The listing builds one solid part. Answer for the finished solid, in the listing's coordinates (mm). A direction names the side the tool comes from. Coordinates: 2 decimals unless noted, no trailing zeros. Write each loop counter-clockwise with the first axis right and the second up, starting at its lowest first coordinate (ties: lowest second). Pieces come first, ordered by that corner, then holes.
```python
from build123d import *

# Parameters (mm, degrees)
SKETCH1_R           = 10
BOSS_EXTRUDE1_DEPTH = 10
SKETCH2_R           = 7.5
BOSS_EXTRUDE2_DEPTH = 10
SKETCH3_R           = 1.5
BOSS_EXTRUDE5_DEPTH = 3
SKETCH7_W           = 1
SKETCH7_H           = 5.758644492
BOSS_EXTRUDE7_DEPTH = 1.5
SKETCH8_R           = 3.25
BOSS_EXTRUDE8_DEPTH = 6.5
BOSS_EXTRUDE9_START = 10
SKETCH9_R           = 1.5
BOSS_EXTRUDE9_DEPTH = 10
FILLET2_SIZE        = 1


with BuildPart() as part:
    # Sketch1 → Boss-Extrude1 (new body)
    with BuildSketch(Plane.XY):
        Circle(SKETCH1_R)
    extrude(amount=BOSS_EXTRUDE1_DEPTH)

    # Sketch2 → Boss-Extrude2 (add)
    with BuildSketch(Plane(origin=(0, 0, 0), x_dir=(-1, 0, 0), z_dir=(0, 0, -1))):
        with Locations(Location((0, 0, 0), (0, 0, 180))):
            Circle(SKETCH2_R)
    extrude(amount=BOSS_EXTRUDE2_DEPTH)

    # Sketch3 → Boss-Extrude5 (add)
    with BuildSketch(Plane(origin=(0, 0, -10), x_dir=(-1, 0, 0), z_dir=(0, 0, -1))):
        Circle(SKETCH3_R)
    extrude(amount=BOSS_EXTRUDE5_DEPTH)

    # Sketch7 → Boss-Extrude7 (add)
    with BuildSketch(Plane(origin=(0, 0, -10), x_dir=(-1, 0, 0), z_dir=(0, 0, -1))):
        with Locations((-5, 0)):
            Rectangle(SKETCH7_W, SKETCH7_H)
        with Locations((5, 0)):
            Rectangle(SKETCH7_W, SKETCH7_H)
    extrude(amount=BOSS_EXTRUDE7_DEPTH)

    # Sketch8 → Boss-Extrude8 (add)
    with BuildSketch(Plane.XY.offset(10)):
        with Locations(Location((0, 0, 0), (0, 0, 180))):
            Circle(SKETCH8_R)
    extrude(amount=BOSS_EXTRUDE8_DEPTH)

    # Sketch9 → Boss-Extrude9 (add)
    with BuildSketch(Plane.XY.offset(16.5).offset(BOSS_EXTRUDE9_START)):
        with Locations(Location((0, 0, 0), (0, 0, 180))):
            Circle(SKETCH9_R)
    extrude(amount=-BOSS_EXTRUDE9_DEPTH)

    # Fillet2
    # a fillet whose section is not a circle: 1 mm, written as the material it takes off along each edge
    with BuildSketch(Plane(origin=(0, 0, 10), x_dir=(1, 0, 0), z_dir=(0, -1, 0))) as fillet2_piece_1:
        with BuildLine():
            Bezier((10, -FILLET2_SIZE), (10, 0), (10 - FILLET2_SIZE, 0), weights=[1, 1, 1])
            Line((10 - FILLET2_SIZE, 0), (10, 0))
            Line((10, 0), (10, -FILLET2_SIZE))
        make_face()
    revolve(axis=Axis((0, 0, 10), (0, 0, 1)), mode=Mode.SUBTRACT)


solid = part.part
```
(1) Section A-A, the plane z = -8.5 is taken. Write down the section's boundary in (x, y).
(2) For a pull along X with two mould halves and no side action, classify faces 1 (the cylindrical face through (4.032, -6.324, -4.93)), 2 (the cylindrical face through (1.5, 0.07, -11.48)), 3 (the flat face through (-5, -2.879, -11)) as pulls with the +X half, pulls with the -X half, needs draft (parallel to the pull), parting line crosses it, or undercut.
(3) Section B-B, the plane z = 7.5 is taken. Write down the section's boundary in (x, y).
(4) Which of the six approach directions +Z, -Z, +X, -X, +Y, -Y give full straight-line access (tool end or side, diameter ignored) to faces 4 (the flat face through (-5.5, 0, -11)), 5 (the flat face through (5.5, 0, -11)), 6 (the flat face through (5, -2.879, -11)), 7 (the flat face through (4, 7, 0))?
(5) Find the intervals of material crossed by probe 1 along Z at (x, y) = (-2.5, 5.75); probe 2 along Z at (x, y) = (-8.5, 0.5); probe 3 along Y at (x, z) = (0, 22), in increasing order.
(6) Each of these flat-tipped pins is pushed along its axis until it touches: pin 1 (6 mm diameter, centred on y = 4, z = 1.5, fed in from +X); pin 2 (0.8 mm diameter, centred on x = 5, z = -11, fed in from -Y); pin 3 (1.1 mm diameter, centred on x = 5, y = -0.5, fed in from -Z); pin 4 (3 mm diameter, centred on x = 4, z = 18.5, fed in from +Y). Where does it stop, or does it pass through?
Solution:
1. outline: circle Ø15 at (0, 0)
2. face 1: parting line crosses it
2. face 2: undercut
2. face 3: needs draft
3. outline: circle Ø20 at (0, 0)
4. face 4: -Z, -X, +Y, -Y
4. face 5: -Z, +X, +Y, -Y
4. face 6: -Z, +X, -X, -Y
4. face 7: -Z
5. probe 1: z = -10 to 10
5. probe 2: z = 0 to 10
5. probe 3: y = -1.5 to 1.5
6. pin 1: stops at x = 9.95
6. pin 2: stops at y = -2.88
6. pin 3: stops at z = -11.5
6. pin 4: passes through
